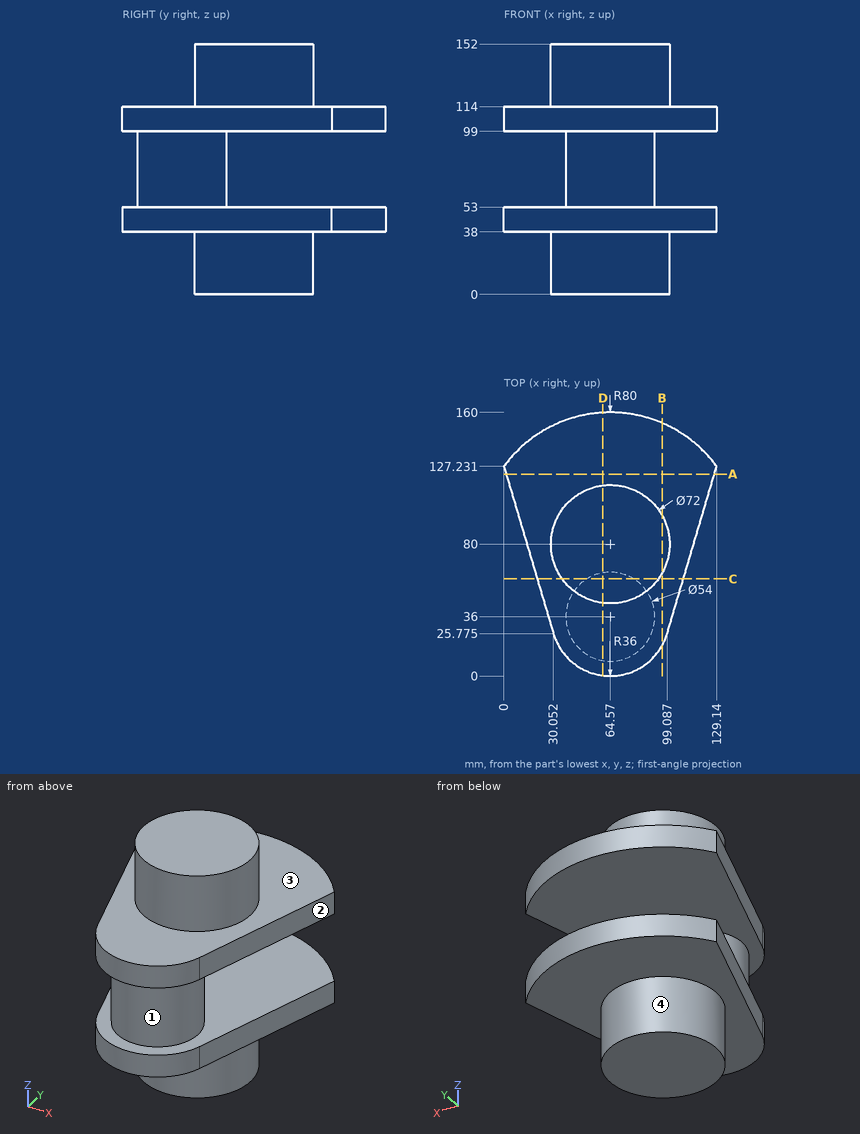
Could you check a few things on this drawing? It's one solid part, dimensions in mm from its lowest x, y, z. A direction names the side the tool comes from. Coordinates: 2 decimals unless noted, no trailing zeros. Order: outer loops, then holes, each group sorted by start corner. A loop starts at its lowest first (then second) coordinate and runs counter-clockwise, first axis right, second up. Notation, with made-up numbers: (-33, 27.25) - (-11, 27.25) arc R27 ccw to (-11, 57.25) - close; hole circle Ø1 at (-3, 54.25). An arc over 180 degrees is marked (long way). One line per question, with ' | ' between items. Start each with the question number.
1. If we section it at D-D (x = 60): Write out the boundary of the cut face in (y, z), and give its area (3 significant figures).
2. If we section it at A-A (y = 122.5): Write out the boundary of the cut face in (x, z), and give its area (3 significant figures).
3. If we section it at B-B (x = 96): Write out the boundary of the cut face in (y, z) (1 decimal), and give its area (3 significant figures).
4. Which directions (+Z, -Z, +X, -X, +Y, -Y) give clear straight access to the entire face, cutting with the end or side of a thin tool? Please do the marked faces 1, 2, 3 and 4.
5. If we section it at C-C (y = 59): Write out the boundary of the cut face in (x, z), and give its area (3 significant figures).
6. Please list where these lines run through material, in increasing order: line 1 along Z through (x, y) = (103.5, 83.5); line 2 along Z through (x, y) = (33, 79.5); line 3 along Z through (x, y) = (85, 32). Write a range as [from, to].
7. I'm going to push flat-ended pins straight in: pin 1 Ø5 at (y, z) = (90.5, 20) entering from +X; pin 2 Ø1.5 at (y, z) = (90.5, 48.5) entering from -X; pin 3 Ø8 at (y, z) = (80, 49) entering from -X (1 decimal). Where does each tip first touch, or does it pass through?
Model answer:
1) outline: (0.29, 38) - (44.29, 38) - (44.29, 0) - (115.71, 0) - (115.71, 38) - (159.87, 38) - (159.87, 53) - (62.61, 53) - (62.61, 99) - (159.87, 99) - (159.87, 114) - (115.71, 114) - (115.71, 152) - (44.29, 152) - (44.29, 114) - (0.29, 114) - (0.29, 99) - (9.39, 99) - (9.39, 53) - (0.29, 53) - close | area: 12,700 mm²
2) outline: (1.4, 38) - (127.74, 38) - (127.74, 53) - (1.4, 53) - close; (1.4, 99) - (127.74, 99) - (127.74, 114) - (1.4, 114) - close | area: 3,790 mm²
3) outline: (18.4, 38) - (62.4, 38) - (62.4, 0) - (97.6, 0) - (97.6, 38) - (153.6, 38) - (153.6, 53) - (18.4, 53) - close; (18.4, 99) - (153.6, 99) - (153.6, 114) - (97.6, 114) - (97.6, 152) - (62.4, 152) - (62.4, 114) - (18.4, 114) - close | area: 6,720 mm²
4) face 1: none | face 2: +Z, -Z, +X, -Y | face 3: +Z | face 4: -Z
5) outline: (20.21, 38) - (35.33, 38) - (35.33, 0) - (93.81, 0) - (93.81, 38) - (108.93, 38) - (108.93, 53) - (78.71, 53) - (78.71, 99) - (108.93, 99) - (108.93, 114) - (93.81, 114) - (93.81, 152) - (35.33, 152) - (35.33, 114) - (20.21, 114) - (20.21, 99) - (50.43, 99) - (50.43, 53) - (20.21, 53) - close | area: 8,410 mm²
6) line 1: z = [38, 53], [99, 114] | line 2: z = [0, 53], [99, 152] | line 3: z = [38, 114]
7) pin 1: stops at x = 99.67 | pin 2: stops at x = 10.66 | pin 3: stops at x = 12.8
